```python
from build123d import *

# Parameters (mm, degrees)
Y_KSEKLIK_EKSTR_ZYON1_DEPTH = 500
IZIM2_R                     = 9
KES_EKSTR_ZYON1_DEPTH       = 100
KES_EKSTR_ZYON3_DEPTH       = 150
KES_EKSTR_ZYON4_DEPTH       = 30


with BuildPart() as part:
    # Çizim1 → Yükseklik-Ekstrüzyon1 (new body)
    with BuildSketch(Plane.XY):
        Polygon((0, 0), (80, 0), (80, 50), (75, 50), (75, 5), (5, 5), (5, 50), (0, 50), align=None)
    extrude(amount=Y_KSEKLIK_EKSTR_ZYON1_DEPTH)

    # Çizim2 → Kes-Ekstrüzyon1 (cut)
    with BuildSketch(Plane(origin=(80, 0, 0), x_dir=(0, 0, -1), z_dir=(1, 0, 0))):
        with Locations((-330, 25)):
            Circle(IZIM2_R)
        with Locations((-190, 25)):
            Circle(IZIM2_R)
    extrude(amount=-KES_EKSTR_ZYON1_DEPTH, mode=Mode.SUBTRACT)

    # Çizim4 → Kes-Ekstrüzyon3 (cut)
    with BuildSketch(Plane(origin=(0, 0, 0), x_dir=(-1, 0, 0), z_dir=(0, 0, -1))):
        Polygon((0, 0), (0, 50), (-5, 50), (-5, 5), (-75, 5), (-75, 50), (-80, 50), (-80, 0), align=None)
    extrude(amount=-KES_EKSTR_ZYON3_DEPTH, mode=Mode.SUBTRACT)

    # Çizim5 → Kes-Ekstrüzyon4 (cut)
    with BuildSketch(Plane.XY.offset(500)):
        Polygon((0, 50), (0, 0), (80, 0), (80, 50), (75, 50), (75, 5), (5, 5), (5, 50), align=None)
    extrude(amount=-KES_EKSTR_ZYON4_DEPTH, mode=Mode.SUBTRACT)


solid = part.part
```
Geometry: final body of the model. Coordinates: model frame, mm. A direction names the side the tool comes from. Give positions to 0.01 mm unless a question says otherwise; leave off trailing zeros. Write each loop counter-clockwise with the first axis right and the second up, starting at its lowest first coordinate (ties: lowest second). Pieces come first, ordered by that corner, then holes.
1. Section query A-A, the plane y = 25. Return loops of the section in (x, z), then the cut area to 3 significant figures.
2. Section query D-D, the plane z = 433. Return loops of the section in (x, y), then the cut area to 3 significant figures.
3. Draft query along X for faces 3 (the flat face through (40, 5, 308)), 4 (the flat face through (42.8, 4.7, 470)), 5 (the flat face through (0, 25, 308)). Return one class per face: released by +X, released by -X, zero draft, split by the parting line, or undercut.
4. Line query: probe 1 along X at (y, z) = (31.5, 385.5); probe 2 along Y at (x, z) = (77.05, 330); probe 3 along Y at (x, z) = (13, 222.5). Output: solid intervals per line, ascending.
5. Pin query (flat end, axial travel): P1, Ø4, axis at y = 18, z = 387.5, coming from the -X side; P2, Ø12, axis at x = 34.5, z = 301.5, coming from the +Y side. Return the tip coordinate at first contact, or that it passes through.
6. Section query C-C, the plane y = 46.5. Return loops of the section in (x, z).
7. Reachability of faces 1 (the cylindrical face through (77.535, 21.553, 321.686)), 2 (the flat face through (5, 27, 308)) from +Z, -Z, +X, -X, +Y, -Y: full face, straight path, thin tool, end or side. Return the list, or none.
8. Section query B-B, the plane z = 190. Return loops of the section in (x, y).
Computed:
1. outline: (0, 150) - (5, 150) - (5, 181) - (0, 181) - close; (0, 199) - (5, 199) - (5, 321) - (0, 321) - close; (0, 339) - (5, 339) - (5, 470) - (0, 470) - close; (75, 150) - (80, 150) - (80, 181) - (75, 181) - close; (75, 199) - (80, 199) - (80, 321) - (75, 321) - close; (75, 339) - (80, 339) - (80, 470) - (75, 470) - close
1. area: 2,840 mm2
2. outline: (0, 0) - (80, 0) - (80, 50) - (75, 50) - (75, 5) - (5, 5) - (5, 50) - (0, 50) - close
2. area: 850 mm2
3. face 3: undercut
3. face 4: zero draft
3. face 5: released by -X
4. probe 1: x = 0 to 5, 75 to 80
4. probe 2: y = 0 to 16, 34 to 50
4. probe 3: y = 0 to 5
5. P1: stops at x = 0
5. P2: stops at y = 5
6. outline: (0, 150) - (5, 150) - (5, 470) - (0, 470) - close; (75, 150) - (80, 150) - (80, 470) - (75, 470) - close
7. face 1: +X, -X
7. face 2: +Z, -Z, +Y
8. outline: (0, 0) - (80, 0) - (80, 16) - (75, 16) - (75, 5) - (5, 5) - (5, 16) - (0, 16) - close; (0, 34) - (5, 34) - (5, 50) - (0, 50) - close; (75, 34) - (80, 34) - (80, 50) - (75, 50) - close
